```python
from build123d import *

# Parameters (mm, degrees)
EXTRUDE1_DEPTH     = 300
SKETCH2_R          = 2.15
CUT_EXTRUDE1_DEPTH = 10


with BuildPart() as part:
    # Sketch1 → Extrude1 (new body)
    with BuildSketch(Plane(origin=(0, 0, 0), x_dir=(0, 0, -1), z_dir=(1, 0, 0))):
        with BuildLine():
            Line((-2.104066935, 2.654149118), (-6.339664187, -2.393639124))
            Line((-6.339664187, -2.393639124), (-7.161057992, -2.776661346))
            Line((-7.161057992, -2.776661346), (-7.600420417, -2.776661346))
            Line((-7.600420417, -2.776661346), (-8.100420417, -3.276661346))
            Line((-8.100420417, -3.276661346), (-8.100420417, -7.1268739))
            Line((-8.100420417, -7.1268739), (-8.600420417, -7.6268739))
            Line((-8.600420417, -7.6268739), (-12, -7.6268739))
            Line((-12, -7.6268739), (-12.5, -8.1268739))
            Line((-12.5, -8.1268739), (-13, -7.6268739))
            Line((-13, -7.6268739), (-16.5, -7.6268739))
            Line((-16.5, -7.6268739), (-17, -8.1268739))
            Line((-17, -8.1268739), (-17, -11.6268739))
            Line((-17, -11.6268739), (-16.5, -12.1268739))
            Line((-16.5, -12.1268739), (-5, -12.1268739))
            Line((-5, -12.1268739), (-5, -7.6268739))
            Line((-5, -7.6268739), (5, -7.6268739))
            Line((5, -7.6268739), (5, -12.1268739))
            Line((5, -12.1268739), (16.5, -12.1268739))
            Line((16.5, -12.1268739), (17, -11.6268739))
            Line((17, -11.6268739), (17, -8.1268739))
            Line((17, -8.1268739), (16.5, -7.6268739))
            Line((16.5, -7.6268739), (13, -7.6268739))
            Line((13, -7.6268739), (12.5, -8.1268739))
            Line((12.5, -8.1268739), (12, -7.6268739))
            Line((12, -7.6268739), (8.600420417, -7.6268739))
            Line((8.600420417, -7.6268739), (8.100420417, -7.1268739))
            Line((8.100420417, -7.1268739), (8.100420417, -3.276661346))
            Line((8.100420417, -3.276661346), (7.600420417, -2.776661346))
            Line((7.600420417, -2.776661346), (7.161057992, -2.776661346))
            Line((7.161057992, -2.776661346), (6.339664187, -2.393639124))
            Line((6.339664187, -2.393639124), (2.104066935, 2.654149118))
            ThreePointArc((2.104066935, 2.654149118), (0, 14.2731261), (-2.104066935, 2.654149118))
        make_face()
    extrude(amount=EXTRUDE1_DEPTH)

    # Sketch2 → Cut-Extrude1 (cut)
    with BuildSketch(Plane.XZ.offset(12.1268739)):
        with Locations((32, -12.5)):
            Circle(SKETCH2_R)
        with Locations((8, -12.5)):
            Circle(SKETCH2_R)
        with Locations((32, 12.5)):
            Circle(SKETCH2_R)
        with Locations((8, 12.5)):
            Circle(SKETCH2_R)
    extrude(amount=-CUT_EXTRUDE1_DEPTH, mode=Mode.SUBTRACT)


solid = part.part
```
For this review, take the finished solid that the model builds, in its own axes (mm). A direction names the side the tool comes from. Coordinates: 2 decimals unless noted, no trailing zeros. Order: outer loops, then holes, each group sorted by start corner. A loop starts at its lowest first (then second) coordinate and runs counter-clockwise, first axis right, second up. Notation, with made-up numbers: (71, -4.75) -> (81, -4.75) arc R23 cw to (81, 12.25) -> close; hole circle Ø7 at (20.5, 1.25). An arc over 180 degrees is marked (long way). Use CSV: the item, a comma, the result in double quotes. Start each with the question number.
Item 1: Draft analysis for pull direction Y (two halves, no side actions). For faces 4 (the face through (148, -12.127, 11)), 5 (the face through (147.9, 0.095, -4.252)), 6 (the face through (0, -2, 0)), state which applies: pulls with the +Y half, pulls with the -Y half, needs draft (parallel to the pull), parting line crosses it, or undercut.
Item 2: We need section B-B, the plane y = 10. Give the boundary of the cut face in (x, z).
Item 3: Insertion check: pin 1 (1 mm diameter, centred on x = 156, z = 10.5, fed in from +Y); pin 2 (1.9 mm diameter, centred on x = 219.5, y = -4.5, fed in from +Z); pin 3 (3 mm diameter, centred on x = 121.5, y = -6, fed in from -Z). Each pin has a flat end and moves straight along its axis. Give the tip position at first contact, or say it passes through.
Item 4: For faces 1 (the face through (147.9, 0.17, 4.19)), 2 (the face through (148, -7.627, 0)), 3 (the face through (148, -12.127, -11)), list the 3-axis set-ups (+Z, -Z, +X, -X, +Y, -Y) from which the entire face can be reached by the end or side of a thin tool; tool diameter is ignored.
Item 5: Wall thickness on probe 1 along Z at (x, y) = (32, -9.3); probe 2 along X at (y, z) = (-9.45, 12.5); probe 3 along Z at (x, y) = (161.5, -8.5): over which ranges is each line inside the solid? List them lowest first.
Derived:
1,face 4,"pulls with the -Y half"
1,face 5,"undercut"
1,face 6,"needs draft"
2,outline,"(0, -5.75) -> (300, -5.75) -> (300, 5.75) -> (0, 5.75) -> close"
3,pin 1,"stops at y = -7.63"
3,pin 2,"stops at z = 8.1"
3,pin 3,"stops at z = -8.47"
4,face 1,"+Z, +X, -X"
4,face 2,"+X, -X, -Y"
4,face 3,"+Z, -Z, +X, -X, -Y"
5,probe 1,"z = -17 to -14.65, -10.35 to -5, 5 to 10.35, 14.65 to 17"
5,probe 2,"x = 0 to 5.85, 10.15 to 29.85, 34.15 to 300"
5,probe 3,"z = -17 to -5, 5 to 17"
